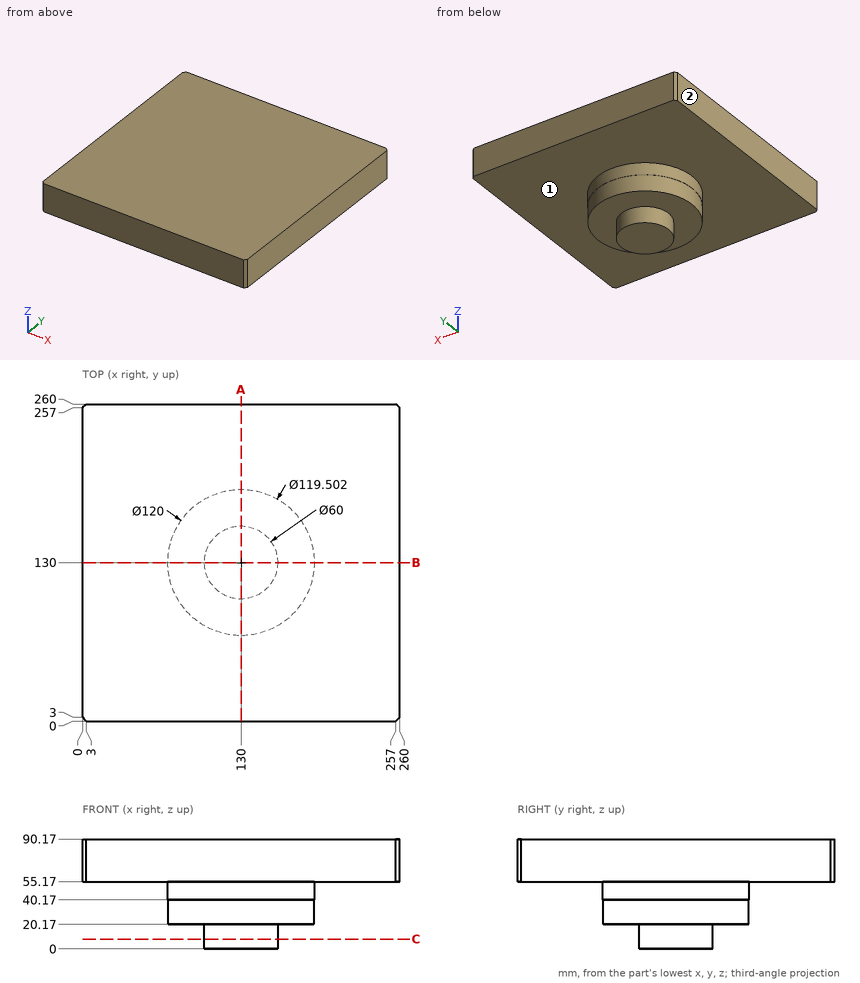
For this review, use the dimensioned drawing (mm, ordinates from the lowest corner) and the shaded views. A direction names the side the tool comes from. Round coordinates to 2 decimals unless told otherwise and drop trailing zeros. Write each loop counter-clockwise with the first axis right and the second up, starting at its lowest first coordinate (ties: lowest second). Pieces come first, ordered by that corner, then holes. Notation, with made-up numbers: (-24.75, 29) - (23.25, 29) arc R22 cw to (23.25, 45) - close; hole circle Ø10 at (8, -7.5). An arc over 180 degrees is marked (long way). Answer as a JSON object with one key per item and string values.
1. Tool access review of the marked faces 1 and 2: name each direction out of +Z, -Z, +X, -X, +Y, -Y from which nothing blocks a thin tool from reaching the whole face with its end or side.
Response values:
{"face 1": "-Z", "face 2": "+Z, -Z, -X, +Y, -Y"}
2. For pin 1 Ø2 at (x, z) = (109, 43) entering from -Y; pin 2 Ø6 at (x, y) = (50, 180) entering from -Z; pin 3 Ø6 at (y, z) = (138, 11.5) entering from +X, all flat-tipped, find the tip position at first contact; note any pin that passes through.
Response values:
{"pin 1": "stops at y = 73.43", "pin 2": "stops at z = 55.17", "pin 3": "stops at x = 159.58"}
3. We need section A-A on x = 130. Give the boundary of the cut face in (y, z).
Response values:
{"outline": "(0, 55.17) - (70, 55.17) - (70, 40.17) - (70.25, 40.17) - (70.25, 20.17) - (100, 20.17) - (100, 0) - (160, 0) - (160, 20.17) - (189.75, 20.17) - (189.75, 40.17) - (190, 40.17) - (190, 55.17) - (260, 55.17) - (260, 90.17) - (0, 90.17) - close"}
4. We need section C-C on z = 8. Give the boundary of the cut face in (x, y).
Response values:
{"outline": "circle Ø60 at (130, 130)"}
5. To check wall thickness, follow line 1 along Z through (x, y) = (16.5, 82); line 2 along Z through (x, y) = (150.5, 86); line 3 along X through (y, z) = (170, 39). State the ranges of each line that lie inside material, in increasing order.
Response values:
{"line 1": "z = 55.17 to 90.17", "line 2": "z = 20.17 to 90.17", "line 3": "x = 85.61 to 174.39"}
